```python
from build123d import *

# Parameters (mm, degrees)
SKETCH1_W           = 70
SKETCH1_H           = 58
BOSS_EXTRUDE1_DEPTH = 3
CHAMFER1_SIZE       = 3


with BuildPart() as part:
    # Sketch1 → Boss-Extrude1 (new body)
    with BuildSketch(Plane.XY):
        with Locations((-125.379084176, 81.977207271)):
            Rectangle(SKETCH1_W, SKETCH1_H)
    extrude(amount=BOSS_EXTRUDE1_DEPTH)

    # Chamfer1
    chamfer1_edges = [part.edges().sort_by_distance(p)[0] for p in [
        (-160.379084176, 81.977207271, 0),
    ]]
    chamfer(chamfer1_edges, length=CHAMFER1_SIZE - 0.0001)  # a hair under: the kernel refuses the full size


solid = part.part
```
Model file for the job. Use its own axes, mm. Round coordinates to 2 decimals unless told otherwise and drop trailing zeros. Order: outer loops, then holes, each group sorted by start corner. A loop starts at its lowest first (then second) coordinate and runs counter-clockwise, first axis right, second up. Notation, with made-up numbers: M -3,62.25 L 27,62.25 A19 cw 27,95.25 Z; hole C 23,-8.5 d11. An arc over 180 degrees is marked long. Use CSV: the item, a comma, the result in double quotes.
Item 1: Saw through at B-B (z = 1.6). List the corners of the cut face in (x, y).
Worked answers:
outline,"M -158.98,52.98 L -90.38,52.98 L -90.38,110.98 L -158.98,110.98 Z"
Item 2: Pull direction Y, two halves, no side cores. Call faces 1 (the face through (-126, 52.977, 1)), 2 (the face through (-158.86, 81.57, 1.48)), 3 (the face through (-126, 110.977, 1)): released by +Y, released by -Y, zero draft, split by the parting line, or undercut.
Worked answers:
face 1,"released by -Y"
face 2,"zero draft"
face 3,"released by +Y"
Item 3: Probe probe 1 along X at (y, z) = (60.5, 0.6); probe 2 along X at (y, z) = (61.5, 1.4). List the from-to ranges inside material, lowest first.
Worked answers:
probe 1,"-157.98 to -90.38"
probe 2,"-158.78 to -90.38"
